Build history of the part. All positions in model axes, mm. Round coordinates to 2 decimals unless told otherwise and drop trailing zeros. Write each loop counter-clockwise with the first axis right and the second up, starting at its lowest first coordinate (ties: lowest second). Pieces come first, ordered by that corner, then holes.
from build123d import *

# Parameters (mm, degrees)
ESBO_O1_R                = 1.5
RESSALTO_EXTRUS_O1_DEPTH = 5.32
FILETE1_R                = 1.5
RESSALTO_EXTRUS_O2_DEPTH = 1
ESBO_O3_W                = 0.5
ESBO_O3_H                = 0.25
RESSALTO_EXTRUS_O3_DEPTH = 2.54
ESBO_O4_W                = 0.93593998
ESBO_O4_H                = 0.492175334
CORTE_EXTRUS_O1_DEPTH    = 1


with BuildPart() as part:
    # Esboço1 → Ressalto-extrusão1 (new body)
    with BuildSketch(Plane.XY):
        Circle(ESBO_O1_R)
    extrude(amount=RESSALTO_EXTRUS_O1_DEPTH)

    # Filete1
    filete1_edges = [part.edges().sort_by_distance(p)[0] for p in [
        (-1.5, 0, 5.32),
    ]]
    fillet(filete1_edges, radius=FILETE1_R)

    # Esboço2 → Ressalto-extrusão2 (add)
    with BuildSketch(Plane(origin=(0, 0, 0), x_dir=(-1, 0, 0), z_dir=(0, 0, -1))):
        with BuildLine():
            Line((1.5, -1.206492851), (1.5, 1.206492851))
            ThreePointArc((1.5, 1.206492851), (-1.925, 0), (1.5, -1.206492851))
        make_face()
    extrude(amount=-RESSALTO_EXTRUS_O2_DEPTH)

    # Esboço3 → Ressalto-extrusão3 (add)
    with BuildSketch(Plane(origin=(0, 0, 0), x_dir=(-1, 0, 0), z_dir=(0, 0, -1))):
        with Locations((-1.3, 0)):
            Rectangle(ESBO_O3_W, ESBO_O3_H)
        with Locations((1.24, 0)):
            Rectangle(ESBO_O3_W, ESBO_O3_H)
    extrude(amount=RESSALTO_EXTRUS_O3_DEPTH)

    # Esboço4 → Corte-extrusão1 (cut)
    with BuildSketch(Plane(origin=(0, 0, -2.54), x_dir=(-1, 0, 0), z_dir=(0, 0, -1))):
        with Locations((1.231752211, 0.012102672)):
            Rectangle(ESBO_O4_W, ESBO_O4_H)
    extrude(amount=-CORTE_EXTRUS_O1_DEPTH, mode=Mode.SUBTRACT)


solid = part.part
1) Wall check: L1, parallel to Y at x = -0.1, z = 0.25; L2, parallel to Y at x = -0.05, z = 3.75; L3, parallel to Z at x = -0.6, y = -1.65. Give the ranges that are in metal, low to high.
Results:
L1: y = -1.92 to 1.92
L2: y = -1.5 to 1.5
L3: z = 0 to 1
2) Slice it at A-A (z = -0.25). Write the cut outline in (x, y) (3 decimals), plus the area to 3 significant figures.
Results:
outline: (-1.49, -0.125) - (-0.99, -0.125) - (-0.99, 0.125) - (-1.49, 0.125) - close; (1.05, -0.125) - (1.55, -0.125) - (1.55, 0.125) - (1.05, 0.125) - close
area: 0.250 mm2
3) Slice it at C-C (y = 0.9). Write the cut outline in (x, z).
Results:
outline: (-1.5, 0) - (1.7, 0) - (1.7, 1) - (1.2, 1) - (1.2, 3.82) arc R1.2 ccw to (-1.2, 3.82) - (-1.2, 1) - (-1.5, 1) - close
4) Slice it at B-B (x = 0). Write the cut outline in (y, z) (3 decimals), plus the area to 3 significant figures.
Results:
outline: (-1.925, 0) - (1.925, 0) - (1.925, 1) - (1.5, 1) - (1.5, 3.82) arc R1.5 ccw to (-1.5, 3.82) - (-1.5, 1) - (-1.925, 1) - close
area: 15.8 mm2
5) Pin check, flat tips, straight feed: pin 1 Ø1.5 at (x, y) = (1, 0.5) entering from -Z; pin 2 Ø1.5 at (y, z) = (1, 4.5) entering from +X; pin 3 Ø0.6 at (x, z) = (-1, -1) entering from -Y (3 decimals). Stop position of each tip, or through.
Results:
pin 1: stops at z = -2.54
pin 2: stops at x = 1.43
pin 3: stops at y = -0.125
6) Slice it at D-D (z = 3). Write the cut outline in (x, y).
Results:
outline: circle Ø3 at (0, 0)
7) Mould opens along Y. For faces 1 (the cylindrical face through (-1.5, 0.07, 2.39)), 2 (the flat face through (-1.5, 0, 0.5)) say: released by +Y, released by -Y, zero draft, split by the parting line, or undercut.
Results:
face 1: split by the parting line
face 2: zero draft
